The listing builds one solid part. Answer for the finished solid, in the listing's coordinates (mm). A direction names the side the tool comes from. Round coordinates to 2 decimals unless told otherwise and drop trailing zeros. Order: outer loops, then holes, each group sorted by start corner. A loop starts at its lowest first (then second) coordinate and runs counter-clockwise, first axis right, second up. Notation, with made-up numbers: (88.25, 29) - (126.25, 29) arc R26 ccw to (126.25, 58) - close; hole circle Ø2 at (-40, 73.5). An arc over 180 degrees is marked (long way). Use CSV: the item, a comma, the result in double quotes. Start each with the question number.
Item 1: Find section D-D, the plane x = 30.5. Give the vertices of the cut face in (y, z), plus the area to 3 significant figures.
Item 2: Flat-ended cylindrical pins translate along their axes: P1, Ø0.6, axis at x = 28, z = 1.5, coming from the +Y side; P2, Ø0.6, axis at y = 35.5, z = 0.5, coming from the -X side; P3, Ø1, axis at y = -32.5, z = 0.5, coming from the +X side. Find the tip coordinate at first contact, or state that the pin passes through.
Item 3: Find section C-C, the plane z = 0.65. Count the separate pieces of the cut face and the enclosed holes in it, plus the area to 3 significant figures.
Item 4: Find section B-B, the plane x = -3. Give the vertices of the cut face in (y, z).
Item 5: Find section A-A, the plane y = -10. Give the vertices of the cut face in (x, z), plus the area to 3 significant figures.
Item 6: Determine the mould class of faces 1 (the flat face through (-28.6, -35.6, 1)), 2 (the cylindrical face through (-76.5, 27.17, 1.01)), 3 (the flat face through (-8, 1, 0)) for opening direction Y: +Y half, -Y half, draft (parallel to the pull), parting line (faces both ways), or undercut.
Item 7: Straight lines are drawn through the part: line 1 along Y through (x, z) = (64, 1.45); line 2 along Y through (x, z) = (52.5, 1.2); line 3 along Y through (x, z) = (-19, 1.35). For each, find the intervals that lie inside material, in ascending order. Write a range as [from, to].
Item 8: For faces 4 (the flat face through (-27.64, 35.39, 0.99)), 5 (the cylindrical face through (-35.26, 20.483, 0.986)), 6 (the cylindrical face through (-83.574, 24.24, 1.014)), determine the directions among +Z, -Z, +X, -X, +Y, -Y from which every point of the face is accessible in a straight line to the end or side of a thin tool.
```python
from build123d import *

# Parameters (mm, degrees)
F0_R        = 4.75
F0_R_2      = 2
F1_DEPTH    = 2
F2_T1_DEPTH = 16.8375789978
F2_T3_DEPTH = 27
F3_R        = 5
F4_R        = 4.99999
F5_R        = 25


# Not quite as in the source:
# - a fillet or chamfer that OpenCascade refuses, or shapes differently, is made with other operations: its cross-section is extruded or revolved along the edge and cut away or added
# - a fillet or chamfer is up to 0.001 mm smaller than in the source, because OpenCascade refuses the exact size


with BuildPart() as f1:
    # F0 (on Top) → F1 (new body)
    with BuildSketch(Plane.XY):
        Polygon((48, -43.5), (67.1863725781, -43.5), (85, -10.8566070522), (85, 10.8566070522), (67.1863725781, 43.5), (48, 43.5), (48, 37.5), (58, 37.5), (58, 27.5), (8, 27.5), (-64.2852836847, 43.5), (-85, 43.5), (-85, 37.5), (-75, 37.5), (-75, 25.7433671504), (-75, 0), (-75, -25.7433671504), (-75, -37.5), (-85, -37.5), (-85, -43.5), (-64.2852836847, -43.5), (8, -27.5), (58, -27.5), (58, -37.5), (48, -37.5), align=None)
        with Locations((64, -10)):
            Circle(F0_R, mode=Mode.SUBTRACT)
        with Locations((-51, 18.5)):
            Circle(F0_R_2, mode=Mode.SUBTRACT)
        with Locations((-35, 18.5)):
            Circle(F0_R_2, mode=Mode.SUBTRACT)
        with Locations((-19, 11.5)):
            Circle(F0_R_2, mode=Mode.SUBTRACT)
        with Locations((-19, 18.5)):
            Circle(F0_R_2, mode=Mode.SUBTRACT)
        with Locations((-19, 25.5)):
            Circle(F0_R_2, mode=Mode.SUBTRACT)
        with Locations((-3, 18.5)):
            Circle(F0_R_2, mode=Mode.SUBTRACT)
        with Locations((72, 0)):
            Circle(F0_R, mode=Mode.SUBTRACT)
        with Locations((64, 10)):
            Circle(F0_R, mode=Mode.SUBTRACT)
        with BuildLine():
            Line((-82.75, 0), (-75, 0))
            Line((-75, 0), (-75, 25.7433671504))
            Line((-75, 25.7433671504), (-85, 15.4460202903))
            Line((-85, 15.4460202903), (-85, 4.0388736054))
            ThreePointArc((-85, 4.0388736054), (-83.3504518318, 2.3116552511), (-82.75, 0))
        make_face()
        with BuildLine():
            Line((-85, 15.4460202903), (-100, 0))
            Line((-100, 0), (-92.25, 0))
            ThreePointArc((-92.25, 0), (-89.8116552511, 4.1495481682), (-85, 4.0388736054))
            Line((-85, 4.0388736054), (-85, 15.4460202903))
        make_face()
        with BuildLine():
            Line((-85, -4.0388736054), (-85, -15.4460202903))
            Line((-85, -15.4460202903), (-75, -25.7433671504))
            Line((-75, -25.7433671504), (-75, 0))
            Line((-75, 0), (-82.75, 0))
            ThreePointArc((-82.75, 0), (-83.3504518318, -2.3116552511), (-85, -4.0388736054))
        make_face()
        with BuildLine():
            Line((-100, 0), (-85, -15.4460202903))
            Line((-85, -15.4460202903), (-85, -4.0388736054))
            ThreePointArc((-85, -4.0388736054), (-89.8116552511, -4.1495481682), (-92.25, 0))
            Line((-92.25, 0), (-100, 0))
        make_face()
        Polygon((-75, 25.7433671504), (-85, 25.7433671504), (-85, 15.4460202903), align=None)
        Polygon((-85, -15.4460202903), (-85, -25.7433671504), (-75, -25.7433671504), align=None)
    extrude(amount=F1_DEPTH)

    # F2: fillet of radius 5 on 10 edges, made by hand

    # F2_s2 → F2_t1 (cut)
    with BuildSketch(Plane.XY.offset(-7.4187894989)):
        with BuildLine():
            ThreePointArc((68.607874454, 40.8951041407), (66.7707657989, 42.7997395679), (64.2188567786, 43.5))
            Line((64.2188567786, 43.5), (67.1863725781, 43.5))
            Line((67.1863725781, 43.5), (68.607874454, 40.8951041407))
        make_face()
        with BuildLine():
            ThreePointArc((64.2188567786, -43.5), (66.7707657989, -42.7997395679), (68.607874454, -40.8951041407))
            Line((68.607874454, -40.8951041407), (67.1863725781, -43.5))
            Line((67.1863725781, -43.5), (64.2188567786, -43.5))
        make_face()
    extrude(amount=F2_T1_DEPTH, mode=Mode.SUBTRACT)

    # F2_s4 → F2_t3 (cut)
    with BuildSketch(Plane.XY.offset(-12.5)):
        with BuildLine():
            ThreePointArc((53, 43.5), (49.4644660941, 42.0355339059), (48, 38.5))
            Line((48, 38.5), (48, 43.5))
            Line((48, 43.5), (53, 43.5))
        make_face()
        with BuildLine():
            ThreePointArc((-85, -38.5), (-83.5355339059, -42.0355339059), (-80, -43.5))
            Line((-80, -43.5), (-85, -43.5))
            Line((-85, -43.5), (-85, -38.5))
        make_face()
        with BuildLine():
            ThreePointArc((-80, -37.5), (-83.5355339059, -38.9644660941), (-85, -42.5))
            Line((-85, -42.5), (-85, -37.5))
            Line((-85, -37.5), (-80, -37.5))
        make_face()
        with BuildLine():
            ThreePointArc((48, -38.5), (49.4644660941, -42.0355339059), (53, -43.5))
            Line((53, -43.5), (48, -43.5))
            Line((48, -43.5), (48, -38.5))
        make_face()
        with BuildLine():
            ThreePointArc((53, -37.5), (49.4644660941, -38.9644660941), (48, -42.5))
            Line((48, -42.5), (48, -37.5))
            Line((48, -37.5), (53, -37.5))
        make_face()
        with BuildLine():
            ThreePointArc((48, 42.5), (49.4644660941, 38.9644660941), (53, 37.5))
            Line((53, 37.5), (48, 37.5))
            Line((48, 37.5), (48, 42.5))
        make_face()
        with BuildLine():
            ThreePointArc((-85, 42.5), (-83.5355339059, 38.9644660941), (-80, 37.5))
            Line((-80, 37.5), (-85, 37.5))
            Line((-85, 37.5), (-85, 42.5))
        make_face()
        with BuildLine():
            ThreePointArc((-80, 43.5), (-83.5355339059, 42.0355339059), (-85, 38.5))
            Line((-85, 38.5), (-85, 43.5))
            Line((-85, 43.5), (-80, 43.5))
        make_face()
    extrude(amount=F2_T3_DEPTH, mode=Mode.SUBTRACT)

    # F3
    f3_edges = [f1.edges().sort_by_distance(p)[0] for p in [
        (58, -27.5, 1),
        (58, 27.5, 1),
    ]]
    fillet(f3_edges, radius=F3_R)

    # F4 (radius 5 in the source; OpenCascade refuses exactly that, so slightly less here)
    f4_edges = [f1.edges().sort_by_distance(p)[0] for p in [
        (-85, 25.743367, 1),
        (-85, -25.743367, 1),
        (-75, 25.743367, 1),
        (-75, -25.743367, 1),
        (-100, 0, 1),
    ]]
    fillet(f4_edges, radius=F4_R)

    # F5
    f5_edges = [f1.edges().sort_by_distance(p)[0] for p in [
        (85, -10.856607, 1),
        (85, 10.856607, 1),
    ]]
    fillet(f5_edges, radius=F5_R)


solid = f1.part
```
Worked out:
1,outline,"(-27.5, 0) - (27.5, 0) - (27.5, 2) - (-27.5, 2) - close"
1,area,"110 mm²"
2,P1,"stops at y = 27.5"
2,P2,"stops at x = -75"
2,P3,"stops at x = 73.46"
3,separate pieces,"1"
3,enclosed holes,"10"
3,area,"11,200 mm²"
4,outline,"(-29.93, 0) - (16.5, 0) - (16.5, 2) - (-29.93, 2) - close; (20.5, 0) - (29.93, 0) - (29.93, 2) - (20.5, 2) - close"
5,outline,"(-90.29, 0) - (59.25, 0) - (59.25, 2) - (-90.29, 2) - close; (68.75, 0) - (84.38, 0) - (84.38, 2) - (68.75, 2) - close"
5,area,"330 mm²"
6,face 1,"-Y half"
6,face 2,"undercut"
6,face 3,"draft"
7,line 1,"y = [-43.5, -14.75], [-5.25, 5.25], [14.75, 43.5]"
7,line 2,"y = [-43.47, -37.53], [-27.5, 27.5], [37.53, 43.47]"
7,line 3,"y = [-33.48, 9.5], [13.5, 16.5], [20.5, 23.5], [27.5, 33.48]"
8,face 4,"+Z, -Z, +Y"
8,face 5,"+Z, -Z"
8,face 6,"+Z, -Z, -X"
